Check sheet for the modelled part. Datum: model origin and axes. Units: mm. A direction names the side the tool comes from. Round coordinates to 2 decimals unless told otherwise and drop trailing zeros. Loops run counter-clockwise (first coordinate to the right, second up) from the corner with the lowest first, then second, coordinate; pieces in that order, holes last. Notation, with made-up numbers: (28.5, 30.5) -> (61.5, 30.5) arc R21 ccw to (61.5, 63.5) -> close; hole circle Ø5 at (80.25, -2). An arc over 180 degrees is marked (long way). One line per question, with ' | ' between items.
```python
from build123d import *

# Parameters (mm, degrees)
SKETCH_1_R          = 20
SKETCH_1_R_2        = 12
EXTRUDE_1_DEPTH     = 25
SKETCH_2_W          = 0.5
SKETCH_2_H          = 19.301562603
CUT_EXTRUDE_1_DEPTH = 15
SKETCH_3_W          = 0.5
SKETCH_3_H          = 20.813345434
CUT_EXTRUDE_2_DEPTH = 15


with BuildPart() as part:
    # 草图1 → 凸台-拉伸1 (new body)
    with BuildSketch(Plane.XY):
        Circle(SKETCH_1_R)
        Circle(SKETCH_1_R_2, mode=Mode.SUBTRACT)
    extrude(amount=EXTRUDE_1_DEPTH)

    # 草图2 → 切除-拉伸1 (cut)
    with BuildSketch(Plane.XY.offset(25)):
        with Locations((-1.434574757, -11.913941214)):
            Rectangle(SKETCH_2_W, SKETCH_2_H)
    extrude(amount=-CUT_EXTRUDE_1_DEPTH, mode=Mode.SUBTRACT)

    # 草图3 → 切除-拉伸2 (cut)
    with BuildSketch(Plane(origin=(0, 0, 0), x_dir=(-1, 0, 0), z_dir=(0, 0, -1))):
        with Locations((-0.669659449, 7.720299062)):
            Rectangle(SKETCH_3_W, SKETCH_3_H)
    extrude(amount=-CUT_EXTRUDE_2_DEPTH, mode=Mode.SUBTRACT)


solid = part.part
```
(1) Scan lines: probe 1 along X at (y, z) = (-0.5, 17); probe 2 along Y at (x, z) = (0, 20.25); probe 3 along Y at (x, z) = (8, 17.25). Record each from-to range of solid material in increasing order.
Answer:
probe 1: x = -19.99 to -11.99, 11.99 to 19.99 | probe 2: y = -20 to -12, 12 to 20 | probe 3: y = -18.33 to -8.94, 8.94 to 18.33
(2) Sectioned sample at B-B, the plane x = 11. Record the cut outline in (y, z), and give its area (3 significant figures).
Answer:
outline: (-16.7, 0) -> (-4.8, 0) -> (-4.8, 25) -> (-16.7, 25) -> close; (4.8, 0) -> (16.7, 0) -> (16.7, 25) -> (4.8, 25) -> close | area: 595 mm2
(3) Sectioned sample at A-A, the plane y = 0. Record the cut outline in (x, z), and give its area (3 significant figures).
Answer:
outline: (-20, 0) -> (-12, 0) -> (-12, 25) -> (-20, 25) -> close; (12, 0) -> (20, 0) -> (20, 25) -> (12, 25) -> close | area: 400 mm2
(4) Sectioned sample at D-D, the plane y = -14. Record the cut outline in (x, z).
Answer:
outline: (-14.28, 0) -> (14.28, 0) -> (14.28, 25) -> (-1.18, 25) -> (-1.18, 10) -> (-1.68, 10) -> (-1.68, 25) -> (-14.28, 25) -> close
(5) Set-up check for faces 4 (the face through (0.42, 15, 7)), 5 (the face through (-1.685, -16, 18)), 6 (the face through (9, -9, 0)): record each of +Z, -Z, +X, -X, +Y, -Y from which the full face is reachable in a straight line by a thin tool's end or side.
Answer:
face 4: -Z | face 5: +Z, -Y | face 6: -Z, +X, -X, +Y, -Y
(6) Mould release check, pull along X, two halves, no side actions. Record for faces 1 (the face through (-4.336, -19.524, 12.325)), 2 (the face through (-1.185, -16, 18)), 3 (the face through (9, -9, 25)): +X half, -X half, draft (parallel to the pull), parting line (faces both ways), or undercut.
Answer:
face 1: parting line | face 2: undercut | face 3: draft
(7) Sectioned sample at C-C, the plane z = 18.25. Record the cut outline in (x, y).
Answer:
outline: (-1.68, -19.93) -> (-1.68, -11.88) arc R12 cw (long way) to (-1.18, -11.94) -> (-1.18, -19.96) arc R20 ccw (long way) to start
(8) Go/stop test with flat-tipped pins: pin 1 (6.5 mm diameter, centred on y = 16, z = 5.5, fed in from +X); pin 2 (4 mm diameter, centred on x = -3, z = 17.5, fed in from -Y) (3 decimals); pin 3 (1 mm diameter, centred on y = -1.5, z = 2.5, fed in from +X) (3 decimals). Record where each tip stops, or that it passes through.
Answer:
pin 1: stops at x = 15.41 | pin 2: stops at y = -19.975 | pin 3: stops at x = 19.975
